```python
from build123d import *

# Parameters (mm, degrees)
SKETCH_R                    = 3.175
BOSS_EXTRUDE1_DEPTH         = 12.7
SKETCH3_W                   = 21.59
SKETCH3_H                   = 17.78
CUT_EXTRUDE1_DEPTH          = 0.762
F_1_4_CLEARANCE_HOLE1_D     = 6.7564
F_1_4_CLEARANCE_HOLE1_DEPTH = 12.7


with BuildPart() as part:
    # Sketch → Boss-Extrude1 (new body)
    with BuildSketch(Plane.XY):
        Polygon((-70.612, 8.89), (32.512, 8.89), (32.512, 0), (32.512, -8.89), (-70.612, -8.89), align=None)
        with Locations((-63.5, 0)):
            Circle(SKETCH_R, mode=Mode.SUBTRACT)
        Circle(SKETCH_R, mode=Mode.SUBTRACT)
        with Locations((25.4, 0)):
            Circle(SKETCH_R, mode=Mode.SUBTRACT)
    extrude(amount=-BOSS_EXTRUDE1_DEPTH)

    # Sketch3 → Cut-Extrude1 (cut)
    with BuildSketch(Plane(origin=(0, 0, 0), x_dir=(-1, 0, 0), z_dir=(0, 0, -1))):
        with Locations((-21.717, 0)):
            Rectangle(SKETCH3_W, SKETCH3_H)
    extrude(amount=CUT_EXTRUDE1_DEPTH, mode=Mode.SUBTRACT)

    # 1/4 Clearance Hole1
    with Locations(Plane.XY):
        with Locations((-50.8, 0), (-12.7, 0)):
            Hole(F_1_4_CLEARANCE_HOLE1_D / 2, depth=F_1_4_CLEARANCE_HOLE1_DEPTH)


solid = part.part
```
For this review, take the finished solid that the model builds, in its own axes (mm). A direction names the side the tool comes from. Round coordinates to 2 decimals unless told otherwise and drop trailing zeros. Write each loop counter-clockwise with the first axis right and the second up, starting at its lowest first coordinate (ties: lowest second). Pieces come first, ordered by that corner, then holes. Notation, with made-up numbers: M 78.5,31 L 111.5,31 A18 ccw 111.5,50 Z; hole C 68,76.5 d3. An arc over 180 degrees is marked long. One line per item, written item: value. Start each with the question number.
(1) Machinability: for faces 4 (the flat face through (22, 0, -0.762)), 5 (the cylindrical face through (-0.69, -3.1, -6.26)), which of the approach directions +Z, -Z, +X, -X, +Y, -Y give a long, thin tool a straight path to every point of the face, cutting with its end or side? Answer none if there is none.
(2) Insertion check: pin 1 (5.5 mm diameter, centred on x = -50.8, y = 0, fed in from -Z); pin 2 (2 mm diameter, centred on x = 21, y = -3.5, fed in from +Z). Each pin has a flat end and moves straight along its axis. Give the tip position at first contact, or say it passes through.
(3) We need section B-B (y = 0). Give the boundary of the cut face in (x, z) (3 decimals), and give its area (3 significant figures).
(4) We need section D-D (x = -50.8). Give the boundary of the cut face in (y, z).
(5) Wall thickness on line 1 (Y direction, x = 0, z = -2.5) (3 decimals); line 2 (Y direction, x = -12.7, z = -10); line 3 (X direction, y = -1.5, z = -10.75): over which ranges is each line inside the solid? List them lowest first.
(6) We need section C-C (z = -5.75). Give the boundary of the cut face in (x, y) (3 decimals), and give its area (3 significant figures).
(7) We need section A-A (x = 25.4). Give the boundary of the cut face in (y, z) (3 decimals), and give its area (3 significant figures).
(8) The part is to be moulded in two halves that separate along X. For faces 1 (the flat face through (-70.612, 0, -6)), 2 (the cylindrical face through (-60.47, 0.95, -6.26)), 3 (the flat face through (-18, -8.89, -6)), say which applies: released by +X, released by -X, zero draft, split by the parting line, or undercut.
Result:
1. face 4: +Z, +X, +Y, -Y
1. face 5: +Z, -Z
2. pin 1: through
2. pin 2: z = -0.76
3. outline: M -70.612,-12.7 L -66.675,-12.7 L -66.675,0 L -70.612,0 Z; M -60.325,-12.7 L -54.178,-12.7 L -54.178,0 L -60.325,0 Z; M -47.422,-12.7 L -16.078,-12.7 L -16.078,0 L -47.422,0 Z; M -9.322,-12.7 L -3.175,-12.7 L -3.175,0 L -9.322,0 Z; M 3.175,-12.7 L 22.225,-12.7 L 22.225,-0.762 L 10.922,-0.762 L 10.922,0 L 3.175,0 Z; M 28.575,-12.7 L 32.512,-12.7 L 32.512,-0.762 L 28.575,-0.762 Z
3. area: 885 mm²
4. outline: M -8.89,-12.7 L -3.38,-12.7 L -3.38,0 L -8.89,0 Z; M 3.38,-12.7 L 8.89,-12.7 L 8.89,0 L 3.38,0 Z
5. line 1: -8.89 to -3.175, 3.175 to 8.89
5. line 2: -8.89 to -3.38, 3.38 to 8.89
5. line 3: -70.61 to -66.3, -60.7 to -53.83, -47.77 to -15.73, -9.67 to -2.8, 2.8 to 22.6, 28.2 to 32.51
6. outline: M -70.612,-8.89 L 32.512,-8.89 L 32.512,8.89 L -70.612,8.89 Z; hole C -63.5,0 d6.35; hole C -50.8,0 d6.756; hole C -12.7,0 d6.756; hole C 0,0 d6.35; hole C 25.4,0 d6.35
6. area: 1,670 mm²
7. outline: M -8.89,-12.7 L -3.175,-12.7 L -3.175,-0.762 L -8.89,-0.762 Z; M 3.175,-12.7 L 8.89,-12.7 L 8.89,-0.762 L 3.175,-0.762 Z
7. area: 136 mm²
8. face 1: released by -X
8. face 2: undercut
8. face 3: zero draft
